Can you work these out from the model? Positions are in its coordinate system, mm. Give positions to 0.01 mm unless a question says otherwise; leave off trailing zeros. Write each loop counter-clockwise with the first axis right and the second up, starting at its lowest first coordinate (ties: lowest second). Pieces come first, ordered by that corner, then holes.
Autodesk Inventor part; units mm, degrees
ref_plane "РабПлоскость2" through (-17.3726, 0, 0) normal (1, 0, 0) x (0, 0, -1)
ref_plane "YZ Plane" through (0, 0, 0) normal (1, 0, 0) x (0, 1, 0)
ref_plane "XZ Plane" through (0, 0, 0) normal (0, 1, 0) x (-1, 0, 0)
sketch "Эскиз1" plane through (0, 0, 0) normal (0, 0, 1) x (1, 0, 0)
  line L0 (0, 0) -> (-17.3726, 0)
  arc A0 (-15, 1.9227) -> (-17, 2.2534) centre (-16.0273, 1.9227) ccw
  line L1 (-15, 1.9227) -> (-15, 1.45)
  line L2 (-15, 1.45) -> (0, 1.45)
  line L3 (0, 1.45) -> (0, 0)
  line L4 (-17.6724, 2.95) -> (-15.1128, 2.95)
  arc A1 (-17, 2.2534) -> (-17.3726, 0) centre (-10.3726, 0) ccw
  dimension "d0" = 2.9
  dimension "d1" = 5.9
  dimension "d2" = 2
  dimension "d3" = 15
  dimension "d4" = 7
revolve "Вращение1" add sketch "Эскиз1" angle 360 about axis through (0, 0, 0) along (-1, 0, 0)
chamfer "Фаска1" distance 0.3 angle 45 1 edges at (0, -1.45, 0)
ref_plane "РабПлоскость2" through (-17.3726, 0, 0) normal (1, 0, 0) x (0, 0, -1)
sketch "Эскиз2" plane through (-17.3726, 0, 0) normal (1, 0, 0) x (0, 0, -1)
  line L0 (-0.4, 1.5) -> (0.4, 1.5)
  line L1 (0.4, 1.5) -> (0.4, -1.5)
  line L2 (0.4, -1.5) -> (-0.4, -1.5)
  line L3 (-0.4, -1.5) -> (-0.4, 1.5)
  line L4 (-1.5, 0.4) -> (1.5, 0.4)
  line L5 (1.5, 0.4) -> (1.5, -0.4)
  line L6 (1.5, -0.4) -> (-1.5, -0.4)
  line L7 (-1.5, -0.4) -> (-1.5, 0.4)
  point P0 (0, 0)
  point P1 (0, 1.5)
  point P2 (0, 0.4)
  point P3 (-1.5, 0)
  point P4 (-0.4, 0)
  point P5 (0.4, 0.4)
  point P6 (-0.4, 0.4)
  point P7 (-0.4, -0.4)
  point P8 (0.4, -0.4)
  dimension "d10" = 0.8
  dimension "d11" = 3
extrude "Выдавливание1" cut sketch "Эскиз2" along normal blind 1.2
properties part number "Винт М3х19"
1) Suppose I cut it at A-A on x = -11. Write out the boundary of the cut face in (y, z), plus the area to 3 significant figures.
Values follow:
outline: circle Ø2.9 at (0, 0)
area: 6.61 mm2
2) For pin 1 Ø0.6 at (x, y) = (-16.5, 0) entering from +Z; pin 2 Ø0.9 at (x, z) = (-17, 1) entering from +Y; pin 3 Ø1.2 at (x, z) = (-16.5, -1) entering from -Y, each with a flat end and sliding along its axis, tell me the tip position at first contact or that it passes through.
Values follow:
pin 1: stops at z = 2.94
pin 2: stops at y = 2.66
pin 3: stops at y = -2.9
3) Please list where these lines run through material, in increasing order: L1, parallel to X at y = -0.15, z = -0.8; L2, parallel to Z at x = -3.5, y = -0.55; L3, parallel to Y at x = -2.75, z = 0.85.
Values follow:
L1: x = -16.17 to 0
L2: z = -1.34 to 1.34
L3: y = -1.17 to 1.17
4) If we mould it in two halves opening along Z, with no side actions, what happens to faces 1 (the face through (0, 0, 0)), 2 (the face through (-17, -1, 0.4)), 3 (the face through (-7.55, -1.45, 0.06))? For each: +Z half, -Z half, draft (parallel to the pull), parting line (faces both ways), or undercut.
Values follow:
face 1: draft
face 2: undercut
face 3: parting line
